from build123d import *

# Parameters (mm, degrees)
SKETCH1_W           = 60.000499048
SKETCH1_H           = 35.031496816
BOSS_EXTRUDE1_DEPTH = 20
SKETCH2_W           = 53.393284908
SKETCH2_H           = 30.292765524
CUT_EXTRUDE1_DEPTH  = 19
SKETCH3_W           = 26.632310578
SKETCH3_H           = 19.17374817
CUT_EXTRUDE2_DEPTH  = 0.5
CUT_EXTRUDE3_DEPTH  = 0.5
SKETCH7_R           = 0.969129223
SKETCH7_R_2         = 0.961352825
CUT_EXTRUDE6_DEPTH  = 5
SKETCH8_R           = 0.104594239
BOSS_EXTRUDE2_DEPTH = 4
SKETCH9_R           = 0.799775616
CUT_EXTRUDE7_DEPTH  = 6
SKETCH10_R          = 1.291760959
CUT_EXTRUDE8_DEPTH  = 0.5
SKETCH13_W          = 13.531174942
SKETCH13_H          = 9.874100633
CUT_EXTRUDE11_DEPTH = 10
SKETCH14_W          = 20.49935166
SKETCH14_H          = 15.002696216
CUT_EXTRUDE12_DEPTH = 1


with BuildPart() as part:
    # Sketch1 → Boss-Extrude1 (new body)
    with BuildSketch(Plane(origin=(0, 0, 0), x_dir=(1, 0, 0), z_dir=(0, 1, 0))):
        Rectangle(SKETCH1_W, SKETCH1_H)
    extrude(amount=BOSS_EXTRUDE1_DEPTH)

    # Sketch2 → Cut-Extrude1 (cut)
    with BuildSketch(Plane(origin=(0, 20, 0), x_dir=(1, 0, 0), z_dir=(0, 1, 0))):
        Rectangle(SKETCH2_W, SKETCH2_H)
    extrude(amount=-CUT_EXTRUDE1_DEPTH, mode=Mode.SUBTRACT)

    # Sketch3 → Cut-Extrude2 (cut)
    with BuildSketch(Plane(origin=(0, 1, 0), x_dir=(1, 0, 0), z_dir=(0, 1, 0))):
        Rectangle(SKETCH3_W, SKETCH3_H)
    extrude(amount=-CUT_EXTRUDE2_DEPTH, mode=Mode.SUBTRACT)

    # Sketch4 → Cut-Extrude3 (cut)
    with BuildSketch(Plane(origin=(0, 0.5, 0), x_dir=(1, 0, 0), z_dir=(0, 1, 0))):
        Polygon((0, -5.07722156), (-12.772700857, -5.07722156), (-12.772700857, 9.032439271), (0, 9.032439271), (12.765065903, 9.032439271), (12.765065903, -5.07722156), align=None)
    extrude(amount=-CUT_EXTRUDE3_DEPTH, mode=Mode.SUBTRACT)

    # Sketch7 → Cut-Extrude6 (cut)
    with BuildSketch(Plane(origin=(0, 20, 0), x_dir=(1, 0, 0), z_dir=(0, 1, 0))):
        with Locations(Location((28.348445989, 0, 0), (0, 0, 270))):
            Circle(SKETCH7_R)
        with Locations(Location((-28.348445989, 0, 0), (0, 0, 270))):
            Circle(SKETCH7_R_2)
    extrude(amount=-CUT_EXTRUDE6_DEPTH, mode=Mode.SUBTRACT)

    # Sketch8 → Boss-Extrude2 (add)
    with BuildSketch(Plane(origin=(0, 20, 0), x_dir=(1, 0, 0), z_dir=(0, 1, 0))):
        with Locations((-28.348445989, 0.961352825)):
            Circle(SKETCH8_R)
        with Locations((-27.51589002, 0.480676413)):
            Circle(SKETCH8_R)
        with Locations((-27.51589002, -0.480676413)):
            Circle(SKETCH8_R)
        with Locations((-28.348445989, -0.961352825)):
            Circle(SKETCH8_R)
        with Locations((-29.181001958, -0.480676413)):
            Circle(SKETCH8_R)
        with Locations((-29.181001958, 0.480676413)):
            Circle(SKETCH8_R)
        with Locations((27.51589002, 0.480676413)):
            Circle(SKETCH8_R)
        with Locations((27.51589002, -0.480676413)):
            Circle(SKETCH8_R)
        with Locations((28.348445989, -0.961352825)):
            Circle(SKETCH8_R)
        with Locations((29.181001958, -0.480676413)):
            Circle(SKETCH8_R)
        with Locations((29.181001958, 0.480676413)):
            Circle(SKETCH8_R)
        with Locations((28.348445989, 0.961352825)):
            Circle(SKETCH8_R)
    extrude(amount=-BOSS_EXTRUDE2_DEPTH)

    # Sketch9 → Cut-Extrude7 (cut)
    with BuildSketch(Plane.XZ):
        with Locations(Location((-21.38647519, 0, 0), (0, 0, 270))):
            Circle(SKETCH9_R)
    extrude(amount=-CUT_EXTRUDE7_DEPTH, mode=Mode.SUBTRACT)

    # Sketch10 → Cut-Extrude8 (cut)
    with BuildSketch(Plane(origin=(0, 1, 0), x_dir=(1, 0, 0), z_dir=(0, 1, 0))):
        with Locations(Location((-21.38647519, 0, 0), (0, 0, 270))):
            Circle(SKETCH10_R)
    extrude(amount=-CUT_EXTRUDE8_DEPTH, mode=Mode.SUBTRACT)

    # Sketch13 → Cut-Extrude11 (cut)
    with BuildSketch(Plane.XY.offset(17.515748408)):
        with Locations((0, 10.335231811)):
            Rectangle(SKETCH13_W, SKETCH13_H)
    extrude(amount=-CUT_EXTRUDE11_DEPTH, mode=Mode.SUBTRACT)

    # Sketch14 → Cut-Extrude12 (cut)
    with BuildSketch(Plane(origin=(0, 0, 15.146382762), x_dir=(-1, 0, 0), z_dir=(0, 0, -1))):
        with Locations((0, 10.335231812)):
            Rectangle(SKETCH14_W, SKETCH14_H)
    extrude(amount=-CUT_EXTRUDE12_DEPTH, mode=Mode.SUBTRACT)


solid = part.part
For this review, take the finished solid that the model builds, in its own axes (mm). A direction names the side the tool comes from. Coordinates: 2 decimals unless noted, no trailing zeros. Write each loop counter-clockwise with the first axis right and the second up, starting at its lowest first coordinate (ties: lowest second). Pieces come first, ordered by that corner, then holes. Notation, with made-up numbers: (35.25, 54.25) -> (45.25, 54.25) arc R10 cw to (45.25, 62.25) -> close; hole circle Ø1 at (-28.75, 54.25). An arc over 180 degrees is marked (long way). Write each question's results on one line, items separated by ' | '. Start each with the question number.
1) Insertion check: pin 1 (2 mm diameter, centred on x = 4, y = 12.5, fed in from +Z); pin 2 (10 mm diameter, centred on x = 11.5, z = -4, fed in from +Y); pin 3 (2 mm diameter, centred on x = -21.39, z = 0, fed in from +Y). Each pin has a flat end and moves straight along its axis. Give the tip position at first contact, or say it passes through.
2) Wall thickness on L1, parallel to X at y = 16.1, z = 0; L2, parallel to X at y = 0.7, z = 0; L3, parallel to Z at x = -15, y = 2.5: over which ranges is each line inside the solid? List them lowest first. Write a range as [from, to].
3) The part is to be moulded in two halves that separate along Y. For faces 4 (the face through (0, 10, -17.516)), 5 (the face through (0, 15.272, 17)), 6 (the face through (-1, 0.5, 6)), say which applies: +Y half, -Y half, draft (parallel to the pull), parting line (faces both ways), or undercut.
4) Consider section A-A (z = -2.5). Write out the cut boundary in (x, y), plus the area to 3 significant figures.
5) Consider section B-B (y = 12.5). Write out the cut boundary in (x, z), plus the area to 3 significant figures.
6) For faces 1 (the face through (6.766, 10, 17)), 2 (the face through (-5, 20, -16)), 3 (the face through (26.697, 11, 0)), list the 3-axis set-ups (+Z, -Z, +X, -X, +Y, -Y) from which the entire face can be reached by the end or side of a thin tool; tool diameter is ignored.
7) Consider section C-C (z = 10.5). Write out the cut boundary in (x, y).
Geometry says:
1) pin 1: z = -15.15 | pin 2: y = 1 | pin 3: y = 0.5
2) L1: [-30, -29.31], [-27.39, -26.7], [26.7, 27.38], [29.32, 30] | L2: [-30, -22.68], [-20.09, -13.32], [13.32, 30] | L3: [-17.52, -15.15], [15.15, 17.52]
3) face 4: draft | face 5: undercut | face 6: +Y half
4) outline: (-30, 0) -> (-12.77, 0) -> (-12.77, 0.5) -> (-13.32, 0.5) -> (-13.32, 1) -> (-26.7, 1) -> (-26.7, 20) -> (-30, 20) -> close; (12.77, 0) -> (30, 0) -> (30, 20) -> (26.7, 20) -> (26.7, 1) -> (13.32, 1) -> (13.32, 0.5) -> (12.77, 0.5) -> close | area: 159 mm^2
5) outline: (-30, -17.52) -> (30, -17.52) -> (30, 17.52) -> (6.77, 17.52) -> (6.77, 16.15) -> (10.25, 16.15) -> (10.25, 15.15) -> (26.7, 15.15) -> (26.7, -15.15) -> (-26.7, -15.15) -> (-26.7, 15.15) -> (-10.25, 15.15) -> (-10.25, 16.15) -> (-6.77, 16.15) -> (-6.77, 17.52) -> (-30, 17.52) -> close | area: 445 mm^2
6) face 1: +Z | face 2: +Z, -Z, +X, -X, +Y | face 3: +Y
7) outline: (-30, 0) -> (30, 0) -> (30, 20) -> (26.7, 20) -> (26.7, 1) -> (-26.7, 1) -> (-26.7, 20) -> (-30, 20) -> close
